Part model, mm, in its own coordinate system. Face numbers are marked on the shaded views. A direction names the side the tool comes from. Round coordinates to 2 decimals unless told otherwise and drop trailing zeros. Write each loop counter-clockwise with the first axis right and the second up, starting at its lowest first coordinate (ties: lowest second). Pieces come first, ordered by that corner, then holes. Notation, with made-up numbers: M -12,85 L 36,85 A30 cw 36,123 Z; hole C 25,20.5 d1. An arc over 180 degrees is marked long. Use one line per item in the form item = value. Start each with the question number.
Item 1: Flat gauge pins, fed straight in: pin 1 Ø1.5 at (x, y) = (-18, -16.5) entering from +Z; pin 2 Ø3 at (x, z) = (8.5, 59.5) entering from +Y. Where does each tip first touch, or does it go through?
Item 2: Cut at D-D, the plane z = 104.5. Give the cut face in (x, y), then the cut area to 3 significant figures.
Item 3: Cut at C-C, the plane y = 3.5. Give the cut face in (x, z).
Item 4: Probe L1, parallel to Y at x = -35.5, z = 9.5; L2, parallel to X at y = -13, z = 53; L3, parallel to Y at x = -33.5, z = 21.5. List the from-to ranges inside material, lowest first.
Item 5: Which spindle directions (+Z, -Z, +X, -X, +Y, -Y) get a long thin tool onto all of the face, cutting with end or side? Do the marked faces 4 and 5. Say none if no direction does.
Item 6: Mould opens along Z. For the marked faces 1, 2 and 3 say: +Z half, -Z half, draft (parallel to the pull), parting line (faces both ways), or undercut.
Item 7: Cut at B-B, the plane x = 47. Give the cut face in (y, z).
Item 8: Cut at A-A, the plane z = 23.5. Give the cut face in (x, y).
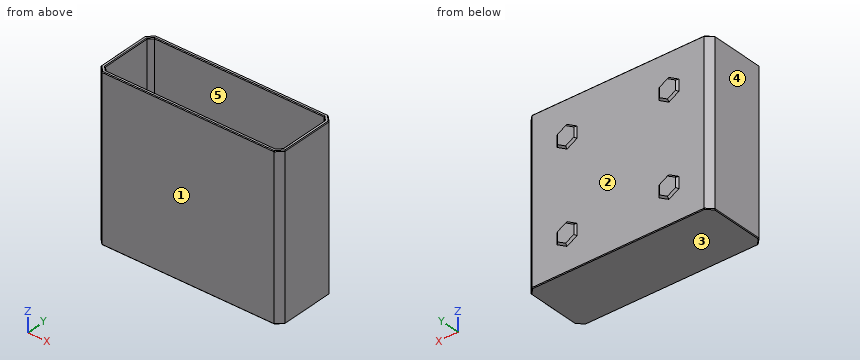
from build123d import *

# Parameters (mm, degrees)
WALLS_DEPTH          = 116.4
BACK_PLATE_DEPTH     = 2
DEBURS_SIZE          = 0.5
FEET_DEPTH           = 1.3
FEET_DRAFT           = -45
FEET_PROFILE_2_DEPTH = 1.3
FEET_PROFILE_2_DRAFT = -45
FEET_PROFILE_3_DEPTH = 1.3
FEET_PROFILE_3_DRAFT = -45
FEET_PROFILE_4_DEPTH = 1.3
FEET_PROFILE_4_DRAFT = -45


with BuildPart() as part:
    # Sketch1 → Walls (new body)
    with BuildSketch(Plane.XY):
        Polygon((-68, 19.535533906), (-68, -19.535533906), (-63.535533906, -24), (63.535533906, -24), (68, -19.535533906), (68, 19.535533906), (63.535533906, 24), (-63.535533906, 24), align=None)
        Polygon((-65.5, 18.5), (-65.5, -18.5), (-62.5, -21.5), (62.5, -21.5), (65.5, -18.5), (65.5, 18.5), (62.5, 21.5), (-62.5, 21.5), align=None, mode=Mode.SUBTRACT)
    extrude(amount=WALLS_DEPTH)

    # Sketch2 → Back Plate (add)
    with BuildSketch(Plane.XY):
        Polygon((68, -19.535533906), (68, 19.535533906), (63.535533906, 24), (-63.535533906, 24), (-68, 19.535533906), (-68, -19.535533906), (-63.535533906, -24), (63.535533906, -24), align=None)
    extrude(amount=-BACK_PLATE_DEPTH)

    # Deburs
    deburs_edges = [part.edges().sort_by_distance(p)[0] for p in [
        (65.5, 0, 0),
        (64, 20, 0),
        (0, 21.5, 0),
        (-64, 20, 0),
        (-65.5, 0, 0),
        (-64, -20, 0),
        (0, -24, 116.4),
        (65.767766953, -21.767766953, 116.4),
        (68, 0, 116.4),
        (65.767766953, -21.767766953, -2),
        (0, -24, -2),
        (-65.767766953, -21.767766953, -2),
        (-68, 0, -2),
        (-65.767766953, 21.767766953, -2),
        (0, 24, -2),
        (65.767766953, 21.767766953, -2),
        (68, 0, -2),
        (65.767766953, 21.767766953, 116.4),
        (0, 24, 116.4),
        (-65.767766953, 21.767766953, 116.4),
        (-68, 0, 116.4),
        (-65.767766953, -21.767766953, 116.4),
        (0, -21.5, 0),
        (0, -21.5, 116.4),
        (-64, -20, 116.4),
        (-65.5, 0, 116.4),
        (-64, 20, 116.4),
        (0, 21.5, 116.4),
        (64, 20, 116.4),
        (65.5, 0, 116.4),
        (64, -20, 116.4),
        (64, -20, 0),
    ]]
    chamfer(deburs_edges, length=DEBURS_SIZE)


with BuildPart() as feet_tool:
    # Sketch4 → Feet (with draft: the straight prism first)
    with BuildSketch(Plane.XZ.offset(-24)):
        Polygon((-30.254771792, 94.633894852), (-37.554771792, 98.848551817), (-44.854771792, 94.633894852), (-44.854771792, 86.204580921), (-37.554771792, 81.989923956), (-30.254771792, 86.204580921), align=None)
    extrude(amount=-FEET_DEPTH)
    # Feet: the draft: its side faces are tilted about the plane it starts from
    feet_sides = [feet_tool.faces().sort_by_distance(p)[0] for p in [
        (-33.904771792, 24.65, 96.741223334),
        (-41.204771792, 24.65, 96.741223334),
        (-44.854771792, 24.65, 90.419237886),
        (-41.204771792, 24.65, 84.097252439),
        (-33.904771792, 24.65, 84.097252439),
        (-30.254771792, 24.65, 90.419237886),
    ]]
    draft(feet_sides, Plane.XZ.offset(-24), FEET_DRAFT)


with BuildPart() as part_1:
    add(part.part)

    # Feet: add feet_tool
    add(feet_tool.part)


with BuildPart() as feet_profile_2_tool:
    # Sketch4 → Feet profile 2 (with draft: the straight prism first)
    with BuildSketch(Plane.XZ.offset(-24)):
        Polygon((-37.554771792, 32.410076044), (-44.854771792, 28.195419079), (-44.854771792, 19.766105148), (-37.554771792, 15.551448183), (-30.254771792, 19.766105148), (-30.254771792, 28.195419079), align=None)
    extrude(amount=-FEET_PROFILE_2_DEPTH)
    # Feet profile 2: the draft: its side faces are tilted about the plane it starts from
    feet_profile_2_sides = [feet_profile_2_tool.faces().sort_by_distance(p)[0] for p in [
        (-41.204771792, 24.65, 30.302747561),
        (-44.854771792, 24.65, 23.980762114),
        (-41.204771792, 24.65, 17.658776666),
        (-33.904771792, 24.65, 17.658776666),
        (-30.254771792, 24.65, 23.980762114),
        (-33.904771792, 24.65, 30.302747561),
    ]]
    draft(feet_profile_2_sides, Plane.XZ.offset(-24), FEET_PROFILE_2_DRAFT)


with BuildPart() as part_2:
    add(part_1.part)

    # Feet profile 2: add feet_profile_2_tool
    add(feet_profile_2_tool.part)


with BuildPart() as feet_profile_3_tool:
    # Sketch4 → Feet profile 3 (with draft: the straight prism first)
    with BuildSketch(Plane.XZ.offset(-24)):
        Polygon((37.554771792, 98.848551817), (30.254771792, 94.633894852), (30.254771792, 86.204580921), (37.554771792, 81.989923956), (44.854771792, 86.204580921), (44.854771792, 94.633894852), align=None)
    extrude(amount=-FEET_PROFILE_3_DEPTH)
    # Feet profile 3: the draft: its side faces are tilted about the plane it starts from
    feet_profile_3_sides = [feet_profile_3_tool.faces().sort_by_distance(p)[0] for p in [
        (33.904771792, 24.65, 96.741223334),
        (30.254771792, 24.65, 90.419237886),
        (33.904771792, 24.65, 84.097252439),
        (41.204771792, 24.65, 84.097252439),
        (44.854771792, 24.65, 90.419237886),
        (41.204771792, 24.65, 96.741223334),
    ]]
    draft(feet_profile_3_sides, Plane.XZ.offset(-24), FEET_PROFILE_3_DRAFT)


with BuildPart() as part_3:
    add(part_2.part)

    # Feet profile 3: add feet_profile_3_tool
    add(feet_profile_3_tool.part)


with BuildPart() as feet_profile_4_tool:
    # Sketch4 → Feet profile 4 (with draft: the straight prism first)
    with BuildSketch(Plane.XZ.offset(-24)):
        Polygon((44.854771792, 19.766105148), (44.854771792, 28.195419079), (37.554771792, 32.410076044), (30.254771792, 28.195419079), (30.254771792, 19.766105148), (37.554771792, 15.551448183), align=None)
    extrude(amount=-FEET_PROFILE_4_DEPTH)
    # Feet profile 4: the draft: its side faces are tilted about the plane it starts from
    feet_profile_4_sides = [feet_profile_4_tool.faces().sort_by_distance(p)[0] for p in [
        (44.854771792, 24.65, 23.980762114),
        (41.204771792, 24.65, 30.302747561),
        (33.904771792, 24.65, 30.302747561),
        (30.254771792, 24.65, 23.980762114),
        (33.904771792, 24.65, 17.658776666),
        (41.204771792, 24.65, 17.658776666),
    ]]
    draft(feet_profile_4_sides, Plane.XZ.offset(-24), FEET_PROFILE_4_DRAFT)


with BuildPart() as part_4:
    add(part_3.part)

    # Feet profile 4: add feet_profile_4_tool
    add(feet_profile_4_tool.part)


solid = part_4.part
Model answer:
q1.pin_1 = 0
q1.pin_2 = 24
q2.outline = M -68,-19.54 L -63.54,-24 L 63.54,-24 L 68,-19.54 L 68,19.54 L 63.54,24 L -63.54,24 L -68,19.54 Z; hole M -65.5,-18.5 L -62.5,-21.5 L 62.5,-21.5 L 65.5,-18.5 L 65.5,18.5 L 62.5,21.5 L -62.5,21.5 L -65.5,18.5 Z
q2.area = 873 mm²
q3.outline = M -68,-1.5 L -67.5,-2 L 67.5,-2 L 68,-1.5 L 68,115.9 L 67.5,116.4 L 66,116.4 L 65.5,115.9 L 65.5,0.5 L 65,0 L -65,0 L -65.5,0.5 L -65.5,115.9 L -66,116.4 L -67.5,116.4 L -68,115.9 Z
q4.L1 = -24 to -21.5, 21.5 to 24
q4.L2 = -68 to -65.5, 65.5 to 68
q4.L3 = -24 to -21.5, 21.5 to 25.3
q5.face_4 = +Z, -Z, -X, +Y, -Y
q5.face_5 = +Z
q6.face_1 = draft
q6.face_2 = undercut
q6.face_3 = -Z half
q7.outline = M -24,-1.5 L -23.5,-2 L 23.5,-2 L 24,-1.5 L 24,115.9 L 23.5,116.4 L 22,116.4 L 21.5,115.9 L 21.5,0.5 L 21,0 L -21,0 L -21.5,0.5 L -21.5,115.9 L -22,116.4 L -23.5,116.4 L -24,115.9 Z
q8.outline = M -68,-19.54 L -63.54,-24 L 63.54,-24 L 68,-19.54 L 68,19.54 L 63.54,24 L 44.85,24 L 43.55,25.3 L 31.55,25.3 L 30.25,24 L -30.25,24 L -31.55,25.3 L -43.55,25.3 L -44.85,24 L -63.54,24 L -68,19.54 Z; hole M -65.5,-18.5 L -62.5,-21.5 L 62.5,-21.5 L 65.5,-18.5 L 65.5,18.5 L 62.5,21.5 L -62.5,21.5 L -65.5,18.5 Z
